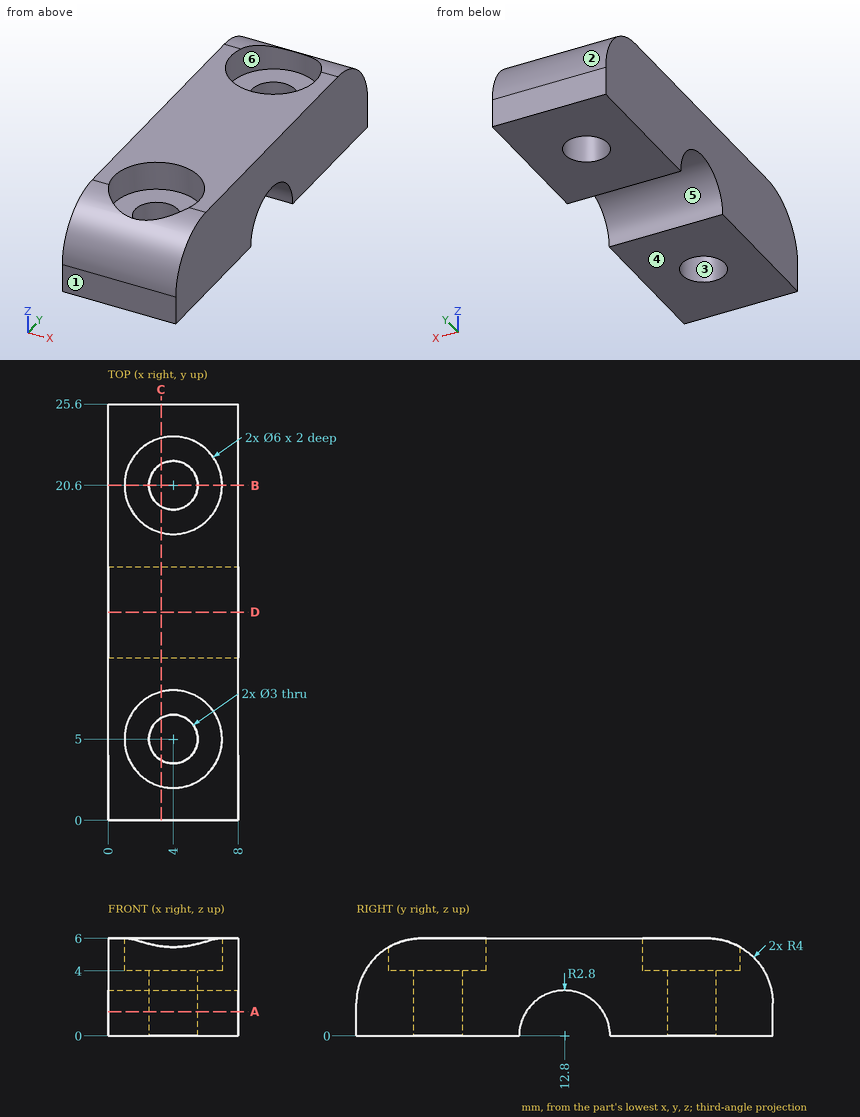
Could you check a few things on this drawing? It's one solid part, dimensions in mm from its lowest x, y, z. A direction names the side the tool comes from. Coordinates: 2 decimals unless noted, no trailing zeros. Loops run counter-clockwise (first coordinate to the right, second up) from the corner with the lowest first, then second, coordinate; pieces in that order, holes last. Notation, with made-up numbers: (78, 46) - (136, 46) arc R17 cw to (136, 68) - close; hole circle Ø10 at (16, 30). An arc over 180 degrees is marked (long way). Answer as a JSON object with one key per item and string values. Group by question number.
Item 1: If I drill on L1, parallel to X at y = 20.75, z = 5.75; L2, parallel to Y at x = 4, z = 4.8; L3, parallel to Z at x = 5.75, y = 4.25, over which ranges is the centre line in solid material (lowest first)? Write a range as from..to.
Item 2: If we mould it in two halves opening along Y, with no side actions, what happens to the marked faces 1, 2, 3 and 4? For each: released by +Y, released by -Y, zero draft, split by the parting line, or undercut.
Item 3: If we section it at C-C (x = 3.25): List the corners of the cut face in (y, z) for me, plus the area to 3 significant figures.
Item 4: On a 3-axis mill with a long thin cutter (end or side, diameter ignored), from which of +Z, -Z, +X, -X, +Y, -Y can I reach the whole of each face in a straight line? I mean the marked faces 5 and 6. Say none if no direction works.
Item 5: If we section it at B-B (y = 20.6): List the corners of the cut face in (x, z) for me.
Item 6: If we section it at D-D (y = 12.8): List the corners of the cut face in (x, z) for me.
Item 7: If we section it at A-A (z = 1.5): List the corners of the cut face in (x, y) for me.
Item 8: For pin 1 (4 mm diameter, centred on x = 1.5, y = 11, fed in from -Z); pin 2 (1.8 mm diameter, centred on x = 5, y = 21, fed in from +Z), each with a flat end and sliding along its axis, tell me the tip position at first contact or that it passes through.
Returned:
{
 "1": {"L1": "x = 0..1, 7..8", "L2": "y = 1.14..2, 8..17.6, 23.6..24.46", "L3": "z = 0..4"},
 "2": {"face 1": "released by -Y", "face 2": "released by +Y", "face 3": "undercut", "face 4": "zero draft"},
 "3": {"outline": "(0, 0) - (3.7, 0) - (3.7, 4) - (2.1, 4) - (2.1, 5.52) arc R4 ccw to (0, 2) - close; (6.3, 0) - (10, 0) arc R2.8 cw to (15.6, 0) - (19.3, 0) - (19.3, 4) - (17.7, 4) - (17.7, 6) - (7.9, 6) - (7.9, 4) - (6.3, 4) - close; (21.9, 0) - (25.6, 0) - (25.6, 2) arc R4 ccw to (23.5, 5.52) - (23.5, 4) - (21.9, 4) - close", "area": "91.0 mm²"},
 "4": {"face 5": "-Z, +X, -X", "face 6": "+Z"},
 "5": {"outline": "(0, 0) - (2.5, 0) - (2.5, 4) - (1, 4) - (1, 6) - (0, 6) - close; (5.5, 0) - (8, 0) - (8, 6) - (7, 6) - (7, 4) - (5.5, 4) - close"},
 "6": {"outline": "(0, 2.8) - (8, 2.8) - (8, 6) - (0, 6) - close"},
 "7": {"outline": "(0, 0) - (8, 0) - (8, 10.44) - (0, 10.44) - close; (0, 15.16) - (8, 15.16) - (8, 25.6) - (0, 25.6) - close; hole circle Ø3 at (4, 5); hole circle Ø3 at (4, 20.6)"},
 "8": {"pin 1": "stops at z = 0", "pin 2": "stops at z = 4"}
}
